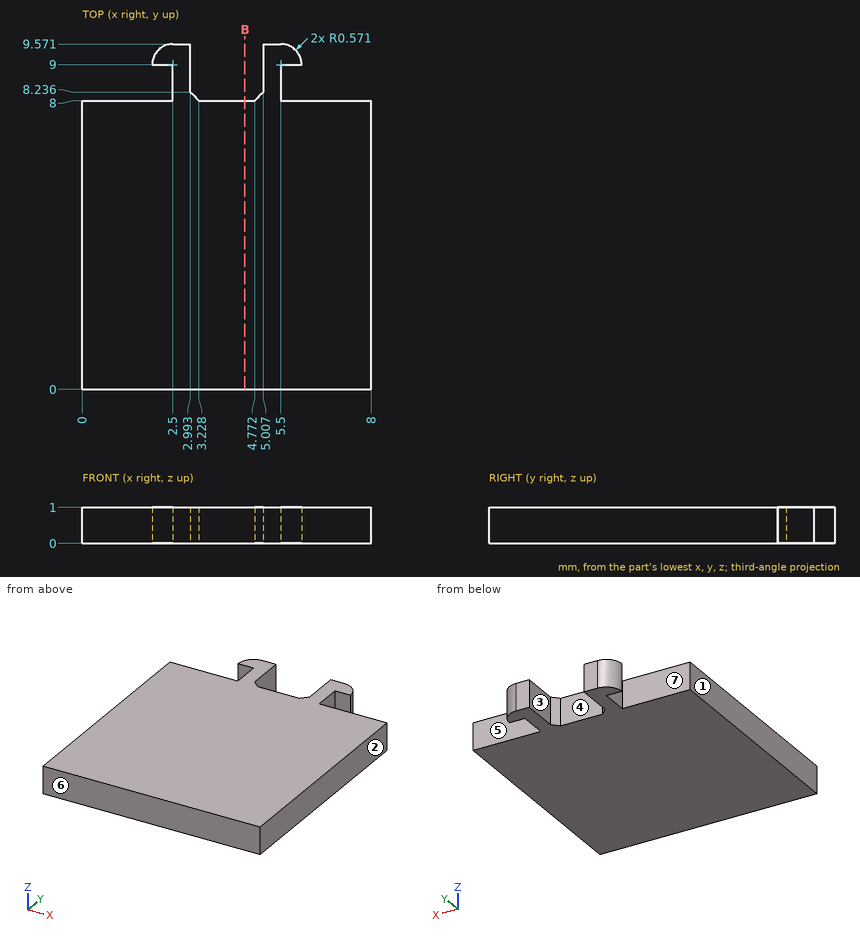
Job drawing, mm, ordinate dimensions from the low corner. One solid piece. A direction names the side the tool comes from. Give positions to 0.01 mm unless a question says otherwise; leave off trailing zeros. Write each loop counter-clockwise with the first axis right and the second up, starting at its lowest first coordinate (ties: lowest second). Pieces come first, ordered by that corner, then holes. Notation, with made-up numbers: M 60.25,82.5 L 68.25,82.5 A13 ccw 68.25,86.5 Z; hole C -35,17 d8. An arc over 180 degrees is marked long. One line per item, written item: value. Start each with the question number.
Q1. Two-plate mould, pull along X, no slides. Class the marked faces 1, 2, 3 and 4: +X half, -X half, draft (parallel to the pull), parting line (faces both ways), or undercut.
Q2. Probe probe 1 along Y at (x, z) = (3.5, 0.3); probe 2 along X at (y, z) = (8.5, 0.9); probe 3 along Y at (x, z) = (2, 0.35) (1 decimal). List the from-to ranges inside material, lowest first. Write a range as [from, to].
Q3. 3-axis set-ups, long thin cutter, end or side, ignore diameter. For the marked faces 5, 6 and 7: which of +Z, -Z, +X, -X, +Y, -Y reach the whole face in a straight line?
Q4. Saw through at B-B, the plane x = 4.5. Write the cut outline in (y, z).
Output values:
1. face 1: -X half
1. face 2: +X half
1. face 3: undercut
1. face 4: undercut
2. probe 1: y = [0, 8]
2. probe 2: x = [2.5, 2.99], [5.01, 5.5]
2. probe 3: y = [0, 8], [9, 9.3]
3. face 5: +Z, -Z, +X
3. face 6: +Z, -Z, +X, -X, -Y
3. face 7: +Z, -Z, -X
4. outline: M 0,0 L 8,0 L 8,1 L 0,1 Z
